```python
from build123d import *

# Parameters (mm, degrees)
SKETCH2_R           = 2
BOSS_EXTRUDE1_DEPTH = 20


with BuildPart() as part:
    # Sketch1 → Revolve1 (revolve)
    with BuildSketch(Plane.XY):
        Polygon((-16.740830618, 1.75), (-1.740830618, 1.75), (28.259169382, 9), (58.259169382, 9), (88.259169382, 1.75), (103.259169382, 1.75), (103.259169382, 0), (-16.740830618, 0), align=None)
    revolve(axis=Axis((103.259169382, 0, 0), (-1, 0, 0)))

    # Sketch2 → Boss-Extrude1 (add)
    with BuildSketch(Plane.XY):
        with Locations(Location((33.259169382, 4, 0), (0, 0, 180))):
            Circle(SKETCH2_R)
        with Locations(Location((33.259169382, -4, 0), (0, 0, 180))):
            Circle(SKETCH2_R)
        with Locations(Location((53.259169382, 4, 0), (0, 0, 180))):
            Circle(SKETCH2_R)
        with Locations(Location((53.259169382, -4, 0), (0, 0, 180))):
            Circle(SKETCH2_R)
    extrude(amount=BOSS_EXTRUDE1_DEPTH)


solid = part.part
```
Could you check a few things on this model? Use its own coordinates, in mm. A direction names the side the tool comes from. Give positions to 0.01 mm unless a question says otherwise; leave off trailing zeros. Loops run counter-clockwise (first coordinate to the right, second up) from the corner with the lowest first, then second, coordinate; pieces in that order, holes last. Notation, with made-up numbers: (-27, 5.25) - (10, 5.25) arc R26 ccw to (10, 23.25) - close; hole circle Ø6 at (52.5, 42.5). An arc over 180 degrees is marked (long way). Answer in a Markdown table with one row per item. Add a question column.
Q1. For pin 1 (10 mm diameter, centred on x = 23, y = 3.5, fed in from +Z); pin 2 (10 mm diameter, centred on x = 3.5, z = 2.5, fed in from -Y); pin 3 (3 mm diameter, centred on x = 13, y = -5, fed in from -Z); pin 4 (2 mm diameter, centred on x = 59, z = 10.5, fed in from -Y), each with a flat end and sliding along its axis, tell me the tip position at first contact or that it passes through.
Q2. We'd pull the mould along X, two halves only. Please class faces 4 (the face through (33.693, 5.952, 13.261)), 5 (the face through (53, 4, 20)), 6 (the face through (13.5, -1.2, 5.3)), 7 (the face through (73.469, -4.225, 3.24)): +X half, -X half, draft (parallel to the pull), parting line (faces both ways), or undercut.
Q3. If we section it at D-D (x = 64): List the corners of the cut face in (y, z) for me.
Q4. Please list where these lines run through material, in increasing order: L1, parallel to X at y = 4, z = 14.25; L2, parallel to X at y = 3.75, z = 10; L3, parallel to Z at x = 19, y = -0.5. Write a range as from..to.
Q5. If we section it at C-C (z = 16.25): List the corners of the cut face in (x, y) for me.
Q6. If we section it at A-A (y = 0): List the corners of the cut face in (x, z) for me.
Q7. Which directions (+Z, -Z, +X, -X, +Y, -Y) give clear straight access to the entire face, cutting with the end or side of a thin tool? Please do faces 1 (the face through (95.864, 1.617, 0.67)), 2 (the face through (53.693, 5.952, 13.261)), 3 (the face through (-9.136, 1.617, 0.67)).
The answers:
| question | item | result |
|---|---|---|
| 1 | pin 1 | stops at z = 8.72 |
| 1 | pin 2 | stops at y = -4.09 |
| 1 | pin 3 | stops at z = -4.08 |
| 1 | pin 4 | passes through |
| 2 | face 4 | undercut |
| 2 | face 5 | draft |
| 2 | face 6 | -X half |
| 2 | face 7 | +X half |
| 3 | outline | circle Ø15.23 at (0, 0) |
| 4 | L1 | x = 31.26..35.26, 51.26..55.26 |
| 4 | L2 | x = 31.27..35.24, 51.27..55.24 |
| 4 | L3 | z = -6.74..6.74 |
| 5 | outline | circle Ø4 at (33.26, -4); circle Ø4 at (33.26, 4); circle Ø4 at (53.26, -4); circle Ø4 at (53.26, 4) |
| 6 | outline | (-16.74, -1.75) - (-1.74, -1.75) - (28.26, -9) - (58.26, -9) - (88.26, -1.75) - (103.26, -1.75) - (103.26, 1.75) - (88.26, 1.75) - (58.26, 9) - (28.26, 9) - (-1.74, 1.75) - (-16.74, 1.75) - close |
| 7 | face 1 | +X |
| 7 | face 2 | +Z |
| 7 | face 3 | -X |
